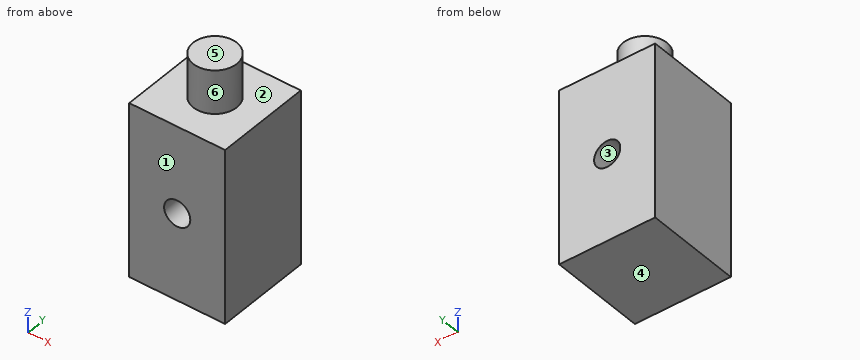
Autodesk Inventor part; units mm, degrees
ref_plane "YZ Plane" through (0, 0, 0) normal (1, 0, 0) x (0, 1, 0)
ref_plane "XZ Plane" through (0, 0, 0) normal (0, 1, 0) x (-1, 0, 0)
ref_plane "XY Plane" through (0, 0, 0) normal (0, 0, 1) x (1, 0, 0)
sketch "Sketch1" plane through (0, 0, 0) normal (0, 0, 1) x (1, 0, 0)
  line L0 (0, 0) -> (11, 0)
  line L1 (11, 0) -> (11, 11)
  line L2 (11, 11) -> (0, 11)
  line L3 (0, 11) -> (0, 0)
  dimension "d0" = 11
  dimension "d1" = 11
extrude "Extrusion1" add sketch "Sketch1" against normal blind 20
sketch "Sketch2" plane through (0, 0, 0) normal (0, 0, 1) x (1, 0, 0)
  line L0 (0, 0) -> (0, 11)
  line L1 (11, 11) -> (11, 0)
  line L2 (0, 11) -> (11, 0)
  line L3 (11, 0) -> (11, 11)
  line L4 (11, 11) -> (0, 0)
  circle A0 centre (5.5, 5.5) radius 2.5
  dimension "d4" = 5
extrude "Extrusion2" add sketch "Sketch2" along normal blind 5 contours A0 L2 L4 | L4 L2 A0 | A0 L4 L2 | L4 A0 L2
sketch "Sketch3" plane through (0, 11, 0) normal (0, 1, 0) x (1, 0, 0)
  line L0 (0, 0) -> (0, 20)
  line L1 (0, 10) -> (11, 10)
  line L2 (11, 0) -> (11, 20)
  line L3 (0, 0) -> (11, 0)
  line L4 (5.5, 0) -> (5.5, 20)
  circle A0 centre (5.5, 10) radius 1.5
  dimension "d7" = 3
extrude "Extrusion3" cut sketch "Sketch3" against normal through all contours A0 L4 L1 | L1 L4 A0 | L4 L1 A0 | L4 A0 L1
properties part number "Aluminium-Connector_Lengan pendek"
Verification items for the finished model (mm, model axes). Face numbers are marked on the shaded views. A direction names the side the tool comes from. Give positions to 0.01 mm unless a question says otherwise; leave off trailing zeros. Loops run counter-clockwise (first coordinate to the right, second up) from the corner with the lowest first, then second, coordinate; pieces in that order, holes last.
1. Set-up check for the marked faces 1 and 2: record each of +Z, -Z, +X, -X, +Y, -Y from which the full face is reachable in a straight line by a thin tool's end or side.
2. Go/stop test with a flat-tipped pin: pin 1 Ø1 at (x, y) = (4, 10) entering from +Z. Record where the tip stops, or that it passes through.
3. Thickness scan on line 1 (Z direction, x = 5.5, y = 4); line 2 (Z direction, x = 9, y = 8); line 3 (X direction, y = 7.5, z = -10). Record the ranges inside material, lowest first.
4. Section check B-B, the plane x = 5.5. Enter the section's corners in (y, z), then the cut area to 3 significant figures.
5. Section check A-A, the plane z = -10. Enter the section's corners in (x, y).
6. Mould release check, pull along Z, two halves, no side actions. Record for the marked faces 3, 4, 5 and 6: released by +Z, released by -Z, zero draft, split by the parting line, or undercut.
7. Section check D-D, the plane y = 5.5. Enter the section's corners in (x, z).
8. Section check C-C, the plane y = 2.75. Enter the section's corners in (x, z).
Geometry says:
1. face 1: +Z, -Z, +X, -X, -Y
1. face 2: +Z
2. pin 1: stops at z = 0
3. line 1: z = -20 to -11.5, -8.5 to 5
3. line 2: z = -20 to 0
3. line 3: x = 0 to 4, 7 to 11
4. outline: (0, -20) - (11, -20) - (11, -11.5) - (0, -11.5) - close; (0, -8.5) - (11, -8.5) - (11, 0) - (8, 0) - (8, 5) - (3, 5) - (3, 0) - (0, 0) - close
4. area: 212 mm2
5. outline: (0, 0) - (4, 0) - (4, 11) - (0, 11) - close; (7, 0) - (11, 0) - (11, 11) - (7, 11) - close
6. face 3: undercut
6. face 4: released by -Z
6. face 5: released by +Z
6. face 6: zero draft
7. outline: (0, -20) - (11, -20) - (11, 0) - (8, 0) - (8, 5) - (3, 5) - (3, 0) - (0, 0) - close; hole circle Ø3 at (5.5, -10)
8. outline: (0, -20) - (11, -20) - (11, 0) - (0, 0) - close; hole circle Ø3 at (5.5, -10)
